```python
from build123d import *
from OCP.BRepFilletAPI import BRepFilletAPI_MakeChamfer

# Parameters (mm, degrees)
SKETCH_1_R          = 55
EXTRUDE_1_DEPTH     = 5
SKETCH_2_R          = 49.9
EXTRUDE_2_DEPTH     = 5
SKETCH_3_W          = 35
SKETCH_3_H          = 45
EXTRUDE_3_DEPTH     = 25
SKETCH_4_W          = 20.2
SKETCH_4_H          = 10.3
CUT_EXTRUDE_1_DEPTH = 99.266220035
SKETCH_5_R          = 4.1
CUT_EXTRUDE_2_DEPTH = 82.700673192
SKETCH_6_R          = 2.75
CUT_EXTRUDE_3_DEPTH = 86.293610546
CHAMFER1_SIZE       = 2
CHAMFER1_SIZE2      = 0.535898385
SKETCH2_W           = 35.065209797
SKETCH2_H           = 45
CUT_EXTRUDE1_DEPTH  = 12.5
BOSS_EXTRUDE1_START = -2
SKETCH4_W           = 70
SKETCH4_H           = 45
BOSS_EXTRUDE1_DEPTH = 5.35
SKETCH5_R           = 4.15
CUT_EXTRUDE2_DEPTH  = 80.281917882
CUT_EXTRUDE3_DEPTH  = 6.5
SKETCH7_W           = 20
SKETCH7_H           = 34
CUT_EXTRUDE4_DEPTH  = 5
CHAMFER2_SIZE       = 1
CHAMFER2_SIZE2      = 2.747477419
SKETCH8_R           = 2.1
CUT_EXTRUDE5_DEPTH  = 79.779756283
CUT_EXTRUDE5_DRAFT  = 2
SKETCH9_W           = 6.2
SKETCH9_H           = 6.2
CUT_EXTRUDE6_DEPTH  = 5
CHAMFER3_SIZE       = 0.7
CHAMFER3_SIZE2      = 2.128636439
SKETCH10_R          = 6
SKETCH10_R_2        = 3
BOSS_EXTRUDE2_DEPTH = 9
FILLET1_R           = 10
FILLET2_R           = 2
SKETCH11_W          = 12.8
SKETCH11_H          = 15
CUT_EXTRUDE7_DEPTH  = 79.779756353
SKETCH13_W          = 10
SKETCH13_H          = 15
CUT_EXTRUDE8_DEPTH  = 4.2


with BuildPart() as part:
    # Эскиз1 → Бобышка-Вытянуть1 (new body)
    with BuildSketch(Plane(origin=(0, 0, 0), x_dir=(1, 0, 0), z_dir=(0, 1, 0))):
        with Locations(Location((0, 0, 0), (0, 0, 270))):
            Circle(SKETCH_1_R)
    extrude(amount=EXTRUDE_1_DEPTH)

    # Эскиз2 → Бобышка-Вытянуть2 (add)
    with BuildSketch(Plane(origin=(0, 5, 0), x_dir=(1, 0, 0), z_dir=(0, 1, 0))):
        with Locations(Location((0, 0, 0), (0, 0, 270))):
            Circle(SKETCH_2_R)
    extrude(amount=EXTRUDE_2_DEPTH)

    # Эскиз3 → Бобышка-Вытянуть3 (add)
    with BuildSketch(Plane.XZ):
        Rectangle(SKETCH_3_W, SKETCH_3_H)
    extrude(amount=EXTRUDE_3_DEPTH)

    # Эскиз4 → Вырез-Вытянуть1 (cut, through all)
    with BuildSketch(Plane.XY.offset(22.5)):
        with Locations((0, -12.5)):
            Rectangle(SKETCH_4_W, SKETCH_4_H)
    extrude(amount=-CUT_EXTRUDE_1_DEPTH, mode=Mode.SUBTRACT)

    # Эскиз5 → Вырез-Вытянуть2 (cut, through all)
    with BuildSketch(Plane.XZ):
        with Locations(Location((33.234018718, -33.234018718, 0), (0, 0, 270))):
            Circle(SKETCH_5_R)
        with Locations(Location((-33.234018718, -33.234018718, 0), (0, 0, 270))):
            Circle(SKETCH_5_R)
        with Locations(Location((-33.234018718, 33.234018718, 0), (0, 0, 270))):
            Circle(SKETCH_5_R)
        with Locations(Location((33.234018718, 33.234018718, 0), (0, 0, 270))):
            Circle(SKETCH_5_R)
    extrude(amount=-CUT_EXTRUDE_2_DEPTH, mode=Mode.SUBTRACT)

    # Эскиз6 → Вырез-Вытянуть3 (cut, through all)
    with BuildSketch(Plane(origin=(0, 10, 0), x_dir=(1, 0, 0), z_dir=(0, 1, 0))):
        with Locations(Location((-18, 28, 0), (0, 0, 270))):
            Circle(SKETCH_6_R)
    extrude(amount=-CUT_EXTRUDE_3_DEPTH, mode=Mode.SUBTRACT)

    # Chamfer1: one chamfer whose edges measure the first distance from different faces: ONE call of the kernel's chamfer builder (chamfer() names one face for all edges)
    chamfer1_edges_1 = [part.edges().sort_by_distance(p)[0] for p in [
        (0, 10, -49.9),
    ]]
    chamfer1_side_1 = [part.faces().sort_by_distance(p)[0] for p in [
        (0, 7.5, -49.9),
    ]]
    chamfer1_edges_2 = [part.edges().sort_by_distance(p)[0] for p in [
        (-49.9, 10, 0),
    ]]
    chamfer1_side_2 = [part.faces().sort_by_distance(p)[0] for p in [
        (-49.9, 7.5, 0),
    ]]
    chamfer1_edges_3 = [part.edges().sort_by_distance(p)[0] for p in [
        (0, 10, 49.9),
    ]]
    chamfer1_side_3 = [part.faces().sort_by_distance(p)[0] for p in [
        (0, 7.5, 49.9),
    ]]
    chamfer1_edges_4 = [part.edges().sort_by_distance(p)[0] for p in [
        (49.9, 10, 0),
    ]]
    chamfer1_side_4 = [part.faces().sort_by_distance(p)[0] for p in [
        (49.9, 7.5, 0),
    ]]
    chamfer1 = BRepFilletAPI_MakeChamfer(part.part.solid().wrapped)
    for e in chamfer1_edges_1:
        chamfer1.Add(CHAMFER1_SIZE, CHAMFER1_SIZE2, e.wrapped, chamfer1_side_1[0].wrapped)  # the first distance lies on this face
    for e in chamfer1_edges_2:
        chamfer1.Add(CHAMFER1_SIZE, CHAMFER1_SIZE2, e.wrapped, chamfer1_side_2[0].wrapped)  # the first distance lies on this face
    for e in chamfer1_edges_3:
        chamfer1.Add(CHAMFER1_SIZE, CHAMFER1_SIZE2, e.wrapped, chamfer1_side_3[0].wrapped)  # the first distance lies on this face
    for e in chamfer1_edges_4:
        chamfer1.Add(CHAMFER1_SIZE, CHAMFER1_SIZE2, e.wrapped, chamfer1_side_4[0].wrapped)  # the first distance lies on this face
    add(Compound.cast(chamfer1.Shape()), mode=Mode.REPLACE)

    # Sketch2 → Cut-Extrude1 (cut)
    with BuildSketch(Plane.XZ.offset(25)):
        with Locations((-0.032604899, 0)):
            Rectangle(SKETCH2_W, SKETCH2_H)
    extrude(amount=-CUT_EXTRUDE1_DEPTH, mode=Mode.SUBTRACT)

    # Sketch4 → Boss-Extrude1 (add)
    with BuildSketch(Plane.XZ.offset(7.35).offset(BOSS_EXTRUDE1_START)):
        Rectangle(SKETCH4_W, SKETCH4_H)
    extrude(amount=-BOSS_EXTRUDE1_DEPTH)

    # Sketch5 → Cut-Extrude2 (cut, through all)
    with BuildSketch(Plane.XZ.offset(5.35)):
        with Locations((25, 15)):
            Circle(SKETCH5_R)
        with Locations((-25, 15)):
            Circle(SKETCH5_R)
        with Locations((25, -15)):
            Circle(SKETCH5_R)
        with Locations((-25, -15)):
            Circle(SKETCH5_R)
    extrude(amount=-CUT_EXTRUDE2_DEPTH, mode=Mode.SUBTRACT)

    # Sketch6 → Cut-Extrude3 (cut)
    with BuildSketch(Plane(origin=(0, 10, 0), x_dir=(1, 0, 0), z_dir=(0, 1, 0))):
        Polygon((-18.504809472, -11.25), (-25, -7.5), (-31.495190528, -11.25), (-31.495190528, -18.75), (-25, -22.5), (-18.504809472, -18.75), align=None)
        Polygon((31.495190528, -11.25), (25, -7.5), (18.504809472, -11.25), (18.504809472, -18.75), (25, -22.5), (31.495190528, -18.75), align=None)
        Polygon((31.495190528, 18.75), (25, 22.5), (18.504809472, 18.75), (18.504809472, 11.25), (25, 7.5), (31.495190528, 11.25), align=None)
        Polygon((-18.504809472, 18.75), (-25, 22.5), (-31.495190528, 18.75), (-31.495190528, 11.25), (-25, 7.5), (-18.504809472, 11.25), align=None)
    extrude(amount=-CUT_EXTRUDE3_DEPTH, mode=Mode.SUBTRACT)

    # Sketch7 → Cut-Extrude4 (cut)
    with BuildSketch(Plane(origin=(0, 10, 0), x_dir=(1, 0, 0), z_dir=(0, 1, 0))):
        Rectangle(SKETCH7_W, SKETCH7_H)
    extrude(amount=-CUT_EXTRUDE4_DEPTH, mode=Mode.SUBTRACT)

    # Chamfer2
    chamfer2_edges = [part.edges().sort_by_distance(p)[0] for p in [
        (-18.504809472, 10, 15),
        (-21.752404736, 10, 9.375),
        (-28.247595264, 10, 9.375),
        (-31.495190528, 10, 15),
        (-28.247595264, 10, 20.625),
        (-21.752404736, 10, 20.625),
        (31.495190528, 10, 15),
        (28.247595264, 10, 9.375),
        (21.752404736, 10, 9.375),
        (18.504809472, 10, 15),
        (21.752404736, 10, 20.625),
        (28.247595264, 10, 20.625),
        (31.495190528, 10, -15),
        (28.247595264, 10, -20.625),
        (21.752404736, 10, -20.625),
        (18.504809472, 10, -15),
        (21.752404736, 10, -9.375),
        (28.247595264, 10, -9.375),
        (-18.504809472, 10, -15),
        (-21.752404736, 10, -20.625),
        (-28.247595264, 10, -20.625),
        (-31.495190528, 10, -15),
        (-28.247595264, 10, -9.375),
        (-21.752404736, 10, -9.375),
    ]]
    chamfer2_side = [part.faces().sort_by_distance(p)[0] for p in [
        (-27.766928677, 10, 32.668824287),
    ]]
    chamfer(chamfer2_edges, length=CHAMFER2_SIZE, length2=CHAMFER2_SIZE2, reference=chamfer2_side[0])


with BuildPart() as cut_extrude5_tool:
    # Sketch8 → Cut-Extrude5 (with draft: the straight prism first)
    with BuildSketch(Plane.XZ):
        with Locations((43, 0)):
            Circle(SKETCH8_R)
    extrude(amount=-CUT_EXTRUDE5_DEPTH)
    # Cut-Extrude5: the draft: its side faces are tilted about the plane it starts from
    cut_extrude5_sides = [cut_extrude5_tool.faces().sort_by_distance(p)[0] for p in [
        (40.9, 39.889878141, 0),
    ]]
    draft(cut_extrude5_sides, Plane.XZ, CUT_EXTRUDE5_DRAFT)


with BuildPart() as part_1:
    add(part.part)

    # Cut-Extrude5: cut by cut_extrude5_tool
    add(cut_extrude5_tool.part, mode=Mode.SUBTRACT)

    # Sketch9 → Cut-Extrude6 (cut)
    with BuildSketch(Plane(origin=(0, 10, 0), x_dir=(1, 0, 0), z_dir=(0, 1, 0))):
        with Locations((43, 0)):
            Rectangle(SKETCH9_W, SKETCH9_H)
    extrude(amount=-CUT_EXTRUDE6_DEPTH, mode=Mode.SUBTRACT)

    # Chamfer3
    chamfer3_edges = [part_1.edges().sort_by_distance(p)[0] for p in [
        (40.725396153, 5, 0),
    ]]
    chamfer3_side = [part_1.faces().sort_by_distance(p)[0] for p in [
        (43, 5, 3.012318759),
    ]]
    chamfer(chamfer3_edges, length=CHAMFER3_SIZE, length2=CHAMFER3_SIZE2, reference=chamfer3_side[0])

    # Sketch10 → Boss-Extrude2 (add)
    with BuildSketch(Plane.XZ):
        with Locations(Location((43, 0, 0), (0, 0, 90))):
            Circle(SKETCH10_R)
        with Locations(Location((43, 0, 0), (0, 0, 270))):
            Circle(SKETCH10_R_2, mode=Mode.SUBTRACT)
    extrude(amount=BOSS_EXTRUDE2_DEPTH)

    # Fillet1
    # the kernel refuses this fillet: 10 mm, written as the material it adds along each edge
    with BuildSketch(Plane(origin=(43, 0, 0), x_dir=(0, 0, 1), z_dir=(1, 0, 0))) as fillet1_piece_1_section:
        with BuildLine():
            CenterArc((15.949874371, 10), FILLET1_R, 185.739170477, 84.260829523)
            Line((6, 9), (5.801002513, 8.98))
            ThreePointArc((5.801002513, 8.98), (5.8, 4.5), (5.8, 0))
            Line((5.8, 0), (6, -0.2))
            Line((6, -0.2), (15.949874371, -0.2))
            Line((15.949874371, -0.2), (15.949874371, 0))
        make_face()
    fillet1_piece_1 = revolve(axis=Axis((43, 0, 0), (0, -1, 0)), mode=Mode.PRIVATE)
    fillet1_piece_1 = fillet1_piece_1 & Plane(origin=(0, -2.503571207, 0), x_dir=(0, 0, 1), z_dir=(0, -1, 0)) * Cylinder(55, 64, mode=Mode.PRIVATE)
    add(fillet1_piece_1)

    # Fillet2
    fillet2_edges = [part_1.edges().sort_by_distance(p)[0] for p in [
        (43, -9, -6),
    ]]
    fillet(fillet2_edges, radius=FILLET2_R)

    # Sketch11 → Cut-Extrude7 (cut, through all)
    with BuildSketch(Plane.XZ):
        with Locations((-19, -32)):
            Rectangle(SKETCH11_W, SKETCH11_H)
        with Locations((-19, 32)):
            Rectangle(SKETCH11_W, SKETCH11_H)
    extrude(amount=-CUT_EXTRUDE7_DEPTH, mode=Mode.SUBTRACT)

    # Sketch13 → Cut-Extrude8 (cut)
    with BuildSketch(Plane(origin=(0, 10, 0), x_dir=(1, 0, 0), z_dir=(0, 1, 0))):
        with Locations((-7.6, 32)):
            Rectangle(SKETCH13_W, SKETCH13_H)
        with Locations((-7.6, -32)):
            Rectangle(SKETCH13_W, SKETCH13_H)
    extrude(amount=-CUT_EXTRUDE8_DEPTH, mode=Mode.SUBTRACT)


solid = part_1.part
```
Check sheet for the modelled part. Datum: model origin and axes. Units: mm. A direction names the side the tool comes from. Round coordinates to 2 decimals unless told otherwise and drop trailing zeros. Write each loop counter-clockwise with the first axis right and the second up, starting at its lowest first coordinate (ties: lowest second). Pieces come first, ordered by that corner, then holes. Notation, with made-up numbers: (45.25, 41.5) -> (51.25, 41.5) arc R25 cw to (51.25, 60.5) -> close; hole circle Ø4 at (-6, -27). An arc over 180 degrees is marked (long way). One line per question, with ' | ' between items. Start each with the question number.
1. Sectioned sample at A-A, the plane x = 0. Record the cut outline in (y, z), then the cut area to 3 significant figures.
2. Depth check by flat-ended pin: pin 1 (2 mm diameter, centred on x = -7, y = 8.5, fed in from +Z); pin 2 (10.5 mm diameter, centred on x = -33.23, z = 33.23, fed in from -Y); pin 3 (1.1 mm diameter, centred on y = 6.5, z = -15, fed in from +X). Enter the tip coordinate at first touch or a pass-through.
3. Sectioned sample at B-B, the plane y = -3. Record the cut outline in (x, z).
4. Scan lines: line 1 along Z through (x, y) = (-25, -2.5); line 2 along X through (y, z) = (4, 34); line 3 along Z through (x, y) = (-13, 1.25). Record each from-to range of solid material in increasing order. Write a range as from..to.
5. Set-up check for faces 5 (the face through (-21.798, 5.403, 20.651)), 6 (the face through (26, -5.35, 0)), 7 (the face through (-25.4, 5, -32)): record each of +Z, -Z, +X, -X, +Y, -Y from which the full face is reachable in a straight line by a thin tool's end or side.
6. Release check for a two-part mould opening along X. For faces 1 (the face through (-17.5, -9, 0)), 2 (the face through (0.502, 9.681, 49.447)), 3 (the face through (21.71, 5.4, -9.4)), 4 (the face through (-14, -12.5, 0)) record: +X half, -X half, draft (parallel to the pull), parting line (faces both ways), or undercut.
Taken from the geometry:
1) outline: (-7.35, -22.5) -> (0, -22.5) -> (0, -55) -> (5, -55) -> (5, -49.9) -> (8, -49.9) -> (10, -49.36) -> (10, -17) -> (5, -17) -> (5, 17) -> (10, 17) -> (10, 49.36) -> (8, 49.9) -> (5, 49.9) -> (5, 55) -> (0, 55) -> (0, 22.5) -> (-7.35, 22.5) -> close | area: 1,210 mm^2
2) pin 1: stops at z = 49.52 | pin 2: stops at y = 0 | pin 3: stops at x = 47.76
3) outline: (-35, -22.5) -> (35, -22.5) -> (35, -3.69) arc R8.81 ccw (long way) to (35, 3.69) -> (35, 22.5) -> (-35, 22.5) -> close; hole circle Ø8.3 at (-25, -15); hole circle Ø8.3 at (-25, 15); hole circle Ø8.3 at (25, -15); hole circle Ø8.3 at (25, 15); hole circle Ø6 at (43, 0)
4) line 1: z = -22.5..-19.15, -10.85..10.85, 19.15..22.5 | line 2: x = -43.23..-37.26, -29.21..-25.4, -12.6..29.21, 37.26..43.23 | line 3: z = -53.44..-39.5, -24.5..24.5, 39.5..53.44
5) face 5: +Y | face 6: +Z, -Z, -Y | face 7: +Y, -Y
6) face 1: -X half | face 2: parting line | face 3: undercut | face 4: draft
